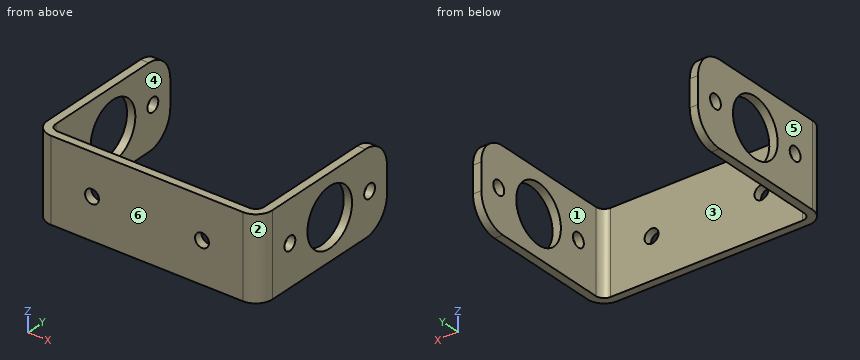
Autodesk Inventor part; units mm, degrees
ref_plane "YZ Plane" through (0, 0, 0) normal (1, 0, 0) x (0, 1, 0)
ref_plane "XZ Plane" through (0, 0, 0) normal (0, 1, 0) x (-1, 0, 0)
ref_plane "XY Plane" through (0, 0, 0) normal (0, 0, 1) x (1, 0, 0)
sketch "Sketch3" plane through (0, 0, 0) normal (0, 1, 0) x (-1, 0, 0)
  line L0 (55, 0) -> (0, 0)
  line L1 (0, 0) -> (0, -20)
  line L2 (0, -20) -> (55, -20)
  line L3 (55, -20) -> (55, 0)
  dimension "d9" = 55
  dimension "d10" = 20
extrude "Plate1" add sketch "Sketch3" along normal blind 2.032
sketch "Sketch4" plane through (-52.968, 0, 0) normal (-1, 0, 0) x (0, -1, 0)
  line L0 (0, -20) -> (0, 0)
  line L1 (0, 0) -> (-40, 0)
  line L2 (-40, 0) -> (-40, -20)
  line L3 (-40, -20) -> (0, -20)
edge flange "Flange1" height 40 angle 90 thickness 2.032 bend radius 2.032 thickness toward (-1, 0, 0) relief tear relief width 2.032 relief depth 1.016 corner gap 2.032 corner form 0 edges at (-55, 2.032, -10) (0, 2.032, -10) wall of the first edge with corners at (-52.968, 0, -20) (-52.968, 0, 0) (-52.968, 40, 0) (-52.968, 40, -20)
bend "Bend1"
corner "Corner1"
sketch "Sketch5" plane through (0, 40, 0) normal (1, 0, 0) x (0, 0, -1)
  line L0 (0, -35.936) -> (20, -35.936)
  line L1 (0, -35.936) -> (20, -35.936)
  line L2 (20, 0) -> (20, -35.936)
  line L3 (0, 0) -> (20, 0)
  line L4 (0, -35.936) -> (0, 0)
  line L5 (20, -35.936) -> (20, 0)
  line L6 (20, -17.968) -> (0, -17.968) construction
  line L7 (0, -35.936) -> (0, 0)
  point P0 (0, -40)
  point P1 (10, -5.468)
  point P2 (10, -17.968)
  point P3 (10, -30.468)
  point P4 (10, -35.936)
  point P5 (10, -17.968)
  dimension "d22" = 12.5
  dimension "d23" = 12.5
hole "Hole1" at (0, 9.532, -10) at (0, 34.532, -10) direction (-1, 0, 0) diameter 3.4 depth 55
hole "Hole2" at (0, 22.032, -10) direction (-1, 0, 0) diameter 14 depth 55
fillet "Fillet1" radius 6.7625 4 edges at (-53.984, 40, 0) (-53.984, 40, -20) (-1.016, 40, -20) (-1.016, 40, 0)
sketch "Sketch6" plane through (0, 2.032, 0) normal (0, 1, 0) x (1, 0, 0)
  line L0 (-4.064, 0) -> (-4.064, 20)
  line L1 (-50.936, 20) -> (-4.064, 20)
  line L2 (-50.936, 20) -> (-50.936, 0)
  line L3 (-4.064, 0) -> (-50.936, 0)
  line L4 (-4.064, 0) -> (-4.064, 20)
  line L5 (-4.064, 10) -> (-14.064, 10) construction
  line L6 (-40.936, 10) -> (-50.936, 10) construction
  point P0 (0, 0)
  dimension "d39" = 10
hole "Hole3" at (-40.936, 2.032, -10) at (-14.064, 2.032, -10) direction (0, -1, 0) diameter 3.4 end through all
equation "\"d29\" = Thickness"
equation "\"d11\" = Thickness"
equation "\"d12\" = BendReliefWidth"
equation "\"d13\" = BendReliefDepth"
equation "\"d14\" = MinimumRemnant"
equation "\"d15\" = TransitionRadius"
equation "\"d18\" = BendRadius"
equation "\"d19\" = CornerReliefSize"
equation "\"d20\" = GapSize"
equation "\"d21\" = JacobiRadiusSize"
equation "\"BendRadius\" = Thickness"
equation "\"BendReliefWidth\" = Thickness"
equation "\"BendReliefDepth\" = 0.5 * Thickness"
equation "\"CornerReliefSize\" = 4 * Thickness"
equation "\"MinimumRemnant\" = 2 * Thickness"
equation "\"TransitionRadius\" = BendRadius"
equation "\"JacobiRadiusSize\" = BendRadius"
equation "\"GapSize\" = Thickness"
properties part number "Flat Pattern"
Can you work these out from the model? Positions are in its coordinate system, mm. Face numbers are marked on the shaded views. A direction names the side the tool comes from. Give positions to 0.01 mm unless a question says otherwise; leave off trailing zeros. Write each loop counter-clockwise with the first axis right and the second up, starting at its lowest first coordinate (ties: lowest second). Pieces come first, ordered by that corner, then holes. Notation, with made-up numbers: (11, -12) -> (53, -12) arc R22 ccw to (53, 4) -> close; hole circle Ø6 at (-4, 84.5). An arc over 180 degrees is marked (long way). Answer as a JSON object with one key per item and string values. Group by question number.
Item 1: Suppose I cut it at D-D (y = 20). Please give me the cut outline in (x, z).
Item 2: For the marked faces 1 and 2, which set-ups out of +Z, -Z, +X, -X, +Y, -Y let a thin tool reach every point of the face, with its end or its side?
Item 3: Suppose I cut it at B-B (z = -15.75). Please give me the cut outline in (x, y), plus the area to 3 significant figures.
Item 4: Suppose I cut it at A-A (y = 6.5). Please give me the cut outline in (x, z).
Item 5: We'd pull the mould along X, two halves only. Please class the marked faces 3, 4, 5 and 6: +X half, -X half, draft (parallel to the pull), parting line (faces both ways), or undercut.
Item 6: Suppose I cut it at C-C (z = -10). State how many separate pieces and enclosed holes the cut face has, plus the area to 3 significant figures.
Item 7: Please list where these lines run through material, in increasing order: line 1 (X direction, y = 4, z = -17.75); line 2 (Y direction, x = -5.5, z = -11); line 3 (X direction, y = 1.1, z = -10). Write a range as [from, to].
Item 8: I'm going to push a flat-ended pin straight in: P1, Ø10, axis at x = -45, z = -3.5, coming from the +Y side. Where does the tip first touch, or does it pass through?
Findings:
{
 "1": {"outline": "(-55, -20) -> (-52.97, -20) -> (-52.97, -16.7) -> (-55, -16.7) -> close; (-55, -3.3) -> (-52.97, -3.3) -> (-52.97, 0) -> (-55, 0) -> close; (-2.03, -20) -> (0, -20) -> (0, -16.7) -> (-2.03, -16.7) -> close; (-2.03, -3.3) -> (0, -3.3) -> (0, 0) -> (-2.03, 0) -> close"},
 "2": {"face 1": "+Z, -Z, +Y", "face 2": "+Z, -Z, +X, -Y"},
 "3": {"outline": "(-55, 4.06) arc R4.06 ccw to (-50.94, 0) -> (-4.06, 0) arc R4.06 ccw to (0, 4.06) -> (0, 18.04) -> (-2.03, 18.04) -> (-2.03, 4.06) arc R2.03 cw to (-4.06, 2.03) -> (-50.94, 2.03) arc R2.03 cw to (-52.97, 4.06) -> (-52.97, 18.04) -> (-55, 18.04) -> close; (-55, 26.02) -> (-52.97, 26.02) -> (-52.97, 39.52) -> (-55, 39.52) -> close; (-2.03, 26.02) -> (0, 26.02) -> (0, 39.52) -> (-2.03, 39.52) -> close", "area": "226 mm²"},
 "4": {"outline": "(-55, -20) -> (-52.97, -20) -> (-52.97, 0) -> (-55, 0) -> close; (-2.03, -20) -> (0, -20) -> (0, 0) -> (-2.03, 0) -> close"},
 "5": {"face 3": "undercut", "face 4": "undercut", "face 5": "-X half", "face 6": "draft"},
 "6": {"separate pieces": "9", "enclosed holes": "0", "area": "162 mm²"},
 "7": {"line 1": "x = [-55, -52.97], [-2.03, 0]", "line 2": "y = [0, 2.03]", "line 3": "x = [-53.72, -42.64], [-39.24, -15.76], [-12.36, -1.28]"},
 "8": {"P1": "stops at y = 2.03"}
}
